```python
from build123d import *

# Parameters (mm, degrees)
SKETCH_1_R          = 14.15
EXTRUDE_1_DEPTH     = 17.1
SKETCH_2_R          = 2.5
EXTRUDE_2_DEPTH     = 13
CHAMFER_1_SIZE      = 3
SKETCH_3_R          = 1.5
CUT_EXTRUDE_1_DEPTH = 4
EXTRUDE_START       = 2
SKETCH_4_R          = 2.5
EXTRUDE_3_DEPTH     = 2


with BuildPart() as part:
    # 草图1 → 凸台-拉伸1 (new body)
    with BuildSketch(Plane(origin=(0, 0, 0), x_dir=(1, 0, 0), z_dir=(0, 1, 0))):
        with Locations(Location((0, 0, 0), (0, 0, 270))):
            Circle(SKETCH_1_R)
    extrude(amount=EXTRUDE_1_DEPTH)

    # 草图2 → 凸台-拉伸2 (add)
    with BuildSketch(Plane(origin=(0, 17.1, 0), x_dir=(1, 0, 0), z_dir=(0, 1, 0))):
        with Locations(Location((0, 0, 0), (0, 0, 90))):
            Circle(SKETCH_2_R)
    extrude(amount=EXTRUDE_2_DEPTH)

    # 倒角1
    chamfer_1_edges = [part.edges().sort_by_distance(p)[0] for p in [
        (0, 0, -14.15),
        (0, 17.1, -14.15),
    ]]
    chamfer(chamfer_1_edges, length=CHAMFER_1_SIZE)

    # 草图3 → 切除-拉伸1 (cut)
    with BuildSketch(Plane.XZ):
        with Locations(Location((-8, 0, 0), (0, 0, 270))):
            Circle(SKETCH_3_R)
        with Locations(Location((0, 8, 0), (0, 0, 270))):
            Circle(SKETCH_3_R)
        with Locations(Location((8, 0, 0), (0, 0, 90))):
            Circle(SKETCH_3_R)
        with Locations(Location((0, -8, 0), (0, 0, 90))):
            Circle(SKETCH_3_R)
    extrude(amount=-CUT_EXTRUDE_1_DEPTH, mode=Mode.SUBTRACT)

    # 草图4 → 凸台-拉伸3 (add)
    with BuildSketch(Plane.XZ.offset(EXTRUDE_START)):
        with Locations(Location((0, 0, 0), (0, 0, 270))):
            Circle(SKETCH_4_R)
    extrude(amount=-EXTRUDE_3_DEPTH)


solid = part.part
```
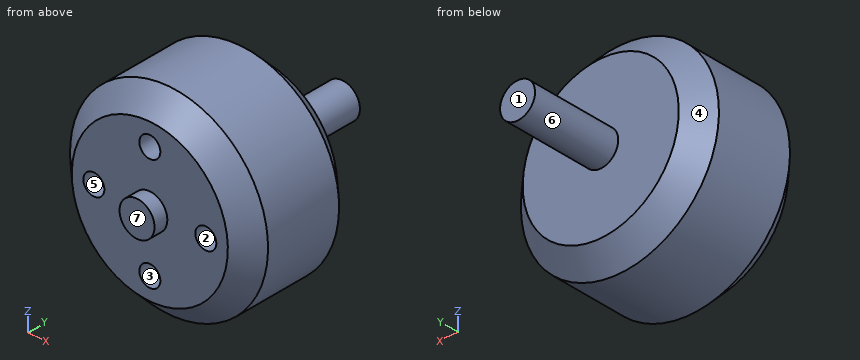
Can you work these out from the model? Positions are in its coordinate system, mm. Face numbers are marked on the shaded views. A direction names the side the tool comes from. Coordinates: 2 decimals unless noted, no trailing zeros. Write each loop counter-clockwise with the first axis right and the second up, starting at its lowest first coordinate (ties: lowest second). Pieces come first, ordered by that corner, then holes. Notation, with made-up numbers: M 27.25,88.25 L 78.25,88.25 A26 cw 78.25,121.25 Z; hole C 85.5,-31.75 d2. An arc over 180 degrees is marked long. Write item = value, one per line. Start each with the question number.
Q1. If I drill on L1, parallel to X at y = 1.6, z = 0; L2, parallel to X at y = 2.5, z = 0; L3, parallel to Y at x = -7.5, z = -5.75, over which ranges is the centre line in solid material (lowest first)? Write a range as [from, to].
Q2. Thinking about a two-plate mould opening in X: for the marked faces 1, 2, 3 and 4, which applies, released by +X, released by -X, zero draft, split by the parting line, or undercut?
Q3. If we section it at B-B, the plane y = 1: Write out the boundary of the cut face in (x, z), then the cut area to 3 significant figures.
Q4. I'm going to push flat-ended pins straight in: pin 1 (3.5 mm diameter, centred on x = -8, z = -0.5, fed in from -Y); pin 2 (2.5 mm diameter, centred on x = 0, z = 8, fed in from +Y); pin 3 (1 mm diameter, centred on x = 10.5, y = 3, fed in from +Z). Where does each tip first touch, or does it pass through?
Q5. If we section it at D-D, the plane y = 24: Write out the boundary of the cut face in (x, z).
Q6. If we section it at A-A, the plane x = 0: Write out the boundary of the cut face in (y, z).
Q7. If we section it at C-C, the plane z = 0: Write out the boundary of the cut face in (x, y).
Q8. On a 3-axis mill with a long thin cutter (end or side, diameter ignored), from which of +Z, -Z, +X, -X, +Y, -Y can I reach the whole of each face in a straight line? I mean the marked faces 5, 6 and 7. Say none if no direction works.
Check sheet entries:
q1.L1 = [-12.75, -9.5], [-6.5, 6.5], [9.5, 12.75]
q1.L2 = [-13.65, -9.5], [-6.5, 6.5], [9.5, 13.65]
q1.L3 = [0, 17.1]
q2.face_1 = zero draft
q2.face_2 = undercut
q2.face_3 = undercut
q2.face_4 = split by the parting line
q3.outline = C 0,0 d24.3; hole C -8,0 d3; hole C 0,-8 d3; hole C 0,8 d3; hole C 8,0 d3
q3.area = 435 mm²
q4.pin_1 = 0
q4.pin_2 = 17.1
q4.pin_3 = 10.01
q5.outline = C 0,0 d5
q6.outline = M -2,-2.5 L 0,-2.5 L 0,-6.5 L 4,-6.5 L 4,-9.5 L 0,-9.5 L 0,-11.15 L 3,-14.15 L 14.1,-14.15 L 17.1,-11.15 L 17.1,-2.5 L 30.1,-2.5 L 30.1,2.5 L 17.1,2.5 L 17.1,11.15 L 14.1,14.15 L 3,14.15 L 0,11.15 L 0,9.5 L 4,9.5 L 4,6.5 L 0,6.5 L 0,2.5 L -2,2.5 Z
q7.outline = M -14.15,3 L -11.15,0 L -9.5,0 L -9.5,4 L -6.5,4 L -6.5,0 L -2.5,0 L -2.5,-2 L 2.5,-2 L 2.5,0 L 6.5,0 L 6.5,4 L 9.5,4 L 9.5,0 L 11.15,0 L 14.15,3 L 14.15,14.1 L 11.15,17.1 L 2.5,17.1 L 2.5,30.1 L -2.5,30.1 L -2.5,17.1 L -11.15,17.1 L -14.15,14.1 Z
q8.face_5 = -Y
q8.face_6 = +Y
q8.face_7 = +Z, -Z, +X, -X, -Y
